```python
from build123d import *

# Parameters (mm, degrees)
CUBE003_W                     = 500
CUBE003_H                     = 500
CUBE003_DEPTH                 = 500
CYLINDER006_R                 = 2.25
CYLINDER006_DEPTH             = 1000
CYLINDER005_R                 = 2.25
CYLINDER005_DEPTH             = 1000
CYLINDER004_R                 = 7.25
CYLINDER004_DEPTH             = 6.5
CYLINDER003_R                 = 7.25
CYLINDER003_DEPTH             = 6.5
GROUP003_PLACEMENT_ANGLE      = 180
CYLINDER002_R                 = 7.25
CYLINDER002_DEPTH             = 6.5
CYLINDER001_R                 = 7.25
CYLINDER001_DEPTH             = 6.5
CYLINDER_R                    = 4
CYLINDER_DEPTH                = 200
CUBE002_W                     = 60
CUBE002_H                     = 21
CUBE002_DEPTH                 = 21
CUBE001_W                     = 30
CUBE001_H                     = 31
CUBE001_DEPTH                 = 26
DIFFERENCE002_PITCH_ANGLE     = 90
DIFFERENCE002_PLACEMENT_ANGLE = 90
REFINELINEAREXTRUDE_R         = 12
REFINELINEAREXTRUDE_R_2       = 1.675
LINEAREXTRUDE_DEPTH           = 20
CUBE_W                        = 42.3
CUBE_H                        = 42.3
CUBE_DEPTH                    = 5
CHAMFER_SIZE                  = 4
CHAMFER001_SIZE               = 1.4
CHAMFER002_SIZE               = 1.4
FILLET_R                      = 5
FILLET001_R                   = 5
FILLET002_R                   = 5
FILLET003_R                   = 5
FILLET004_R                   = 5
FILLET005_R                   = 5


with BuildPart() as cube003:
    # cube003 → cube003 (new body)
    with BuildSketch(Plane(origin=(-250, -510, -250), x_dir=(1, 0, 0), z_dir=(0, 0, 1))):
        with Locations((250, 250)):
            Rectangle(CUBE003_W, CUBE003_H)
    extrude(amount=CUBE003_DEPTH)


with BuildPart() as cylinder006:
    # cylinder006 → cylinder006 (new body)
    with BuildSketch(Plane(origin=(15.5, 500, 0), x_dir=(1, 0, 0), z_dir=(0, -1, 0))):
        Circle(CYLINDER006_R)
    extrude(amount=CYLINDER006_DEPTH)


with BuildPart() as union002:
    # cylinder005 → cylinder005 (new body)
    with BuildSketch(Plane.XZ.offset(-500)):
        Circle(CYLINDER005_R)
    extrude(amount=CYLINDER005_DEPTH)

    # Group005: union cylinder006
    add(cylinder006.part)


with BuildPart() as union002_1:
    # Group005 placement: moved
    add(union002.part.moved(Location((2.25, 0, -15.5))))

    # union002: union cube003
    add(cube003.part)


with BuildPart() as cylinder004:
    # cylinder004 → cylinder004 (new body)
    with BuildSketch(Plane(origin=(15.5, 0, 0), x_dir=(1, 0, 0), z_dir=(0, -1, 0))):
        Circle(CYLINDER004_R)
    extrude(amount=CYLINDER004_DEPTH)


with BuildPart() as group003:
    # cylinder003 → cylinder003 (new body)
    with BuildSketch(Plane.XZ):
        Circle(CYLINDER003_R)
    extrude(amount=CYLINDER003_DEPTH)

    # Group003: union cylinder004
    add(cylinder004.part)


with BuildPart() as group003_1:
    # Group003 placement: moved
    add(group003.part.moved(Location((2.25, 10.5, -15.5))).rotate(Axis((2.25, 10.5, -15.5), (1, 0, 0)), GROUP003_PLACEMENT_ANGLE))


with BuildPart() as cylinder002:
    # cylinder002 → cylinder002 (new body)
    with BuildSketch(Plane(origin=(15.5, 0, 0), x_dir=(1, 0, 0), z_dir=(0, -1, 0))):
        Circle(CYLINDER002_R)
    extrude(amount=CYLINDER002_DEPTH)


with BuildPart() as group004:
    # cylinder001 → cylinder001 (new body)
    with BuildSketch(Plane.XZ):
        Circle(CYLINDER001_R)
    extrude(amount=CYLINDER001_DEPTH)

    # Group002: union cylinder002
    add(cylinder002.part)


with BuildPart() as group004_1:
    # Group002 placement: moved
    add(group004.part.moved(Location((2.25, -10.5, -15.5))))

    # Group004: union Group003
    add(group003_1.part)


with BuildPart() as cylinder:
    # cylinder → cylinder (new body)
    with BuildSketch(Plane(origin=(-100, 15, 13), x_dir=(0, 1, 0), z_dir=(1, 0, 0))):
        Circle(CYLINDER_R)
    extrude(amount=CYLINDER_DEPTH)


with BuildPart() as union:
    # cube002 → cube002 (new body)
    with BuildSketch(Plane(origin=(-30, -10.5, -13), x_dir=(1, 0, 0), z_dir=(0, 0, 1))):
        with Locations((30, 10.5)):
            Rectangle(CUBE002_W, CUBE002_H)
    extrude(amount=CUBE002_DEPTH)

    # union: union cylinder
    add(cylinder.part)


with BuildPart() as difference002:
    # cube001 → cube001 (new body)
    with BuildSketch(Plane(origin=(-15, -15.5, -13), x_dir=(1, 0, 0), z_dir=(0, 0, 1))):
        with Locations((15, 15.5)):
            Rectangle(CUBE001_W, CUBE001_H)
    extrude(amount=CUBE001_DEPTH)

    # difference001: cut union
    add(union.part, mode=Mode.SUBTRACT)


with BuildPart() as difference002_1:
    # difference001 placement: moved
    add(difference002.part.moved(Location((10, 0, -13))))

    # union001: union Group004
    add(group004_1.part)

    # difference002: cut union002
    add(union002_1.part, mode=Mode.SUBTRACT)


with BuildPart() as difference002_2:
    # difference002 pitch: moved
    add(difference002_1.part.rotate(Axis((0, 0, 0), (0, 1, 0)), DIFFERENCE002_PITCH_ANGLE))


with BuildPart() as difference002_3:
    # difference002 placement: moved
    add(difference002_2.part.moved(Location((21.15, 5, 25))).rotate(Axis((21.15, 5, 25), (0, 0, 1)), DIFFERENCE002_PLACEMENT_ANGLE))


with BuildPart() as linearextrude:
    # RefineLinearExtrude → LinearExtrude (new body)
    with BuildSketch(Plane(origin=(0, 0, 0), x_dir=(0, 1, 0), z_dir=(0, 0, 1))):
        Circle(REFINELINEAREXTRUDE_R)
        with Locations((15.5, -15.5)):
            Circle(REFINELINEAREXTRUDE_R_2)
        with Locations((15.5, 15.5)):
            Circle(REFINELINEAREXTRUDE_R_2)
        with Locations((-15.5, 15.5)):
            Circle(REFINELINEAREXTRUDE_R_2)
        with Locations((-15.5, -15.5)):
            Circle(REFINELINEAREXTRUDE_R_2)
    extrude(amount=LINEAREXTRUDE_DEPTH)


with BuildPart() as linearextrude_1:
    # LinearExtrude placement: moved
    add(linearextrude.part.moved(Location((21.15, 21.15, -10))))


with BuildPart() as fillet005:
    # cube → cube (new body)
    with BuildSketch(Plane.XY):
        with Locations((21.15, 21.15)):
            Rectangle(CUBE_W, CUBE_H)
    extrude(amount=CUBE_DEPTH)

    # difference: cut LinearExtrude
    add(linearextrude_1.part, mode=Mode.SUBTRACT)

    # Fusion: union difference002
    add(difference002_3.part)

    # Chamfer
    chamfer_edges = [fillet005.edges().sort_by_distance(p)[0] for p in [
        (20.65, 5, 5),
    ]]
    chamfer(chamfer_edges, length=CHAMFER_SIZE)

    # Chamfer001
    chamfer001_edges = [fillet005.edges().sort_by_distance(p)[0] for p in [
        (4.15, -10.5, 30),
    ]]
    chamfer(chamfer001_edges, length=CHAMFER001_SIZE)

    # Chamfer002
    chamfer002_edges = [fillet005.edges().sort_by_distance(p)[0] for p in [
        (4.15, -10.5, 14.5),
    ]]
    chamfer(chamfer002_edges, length=CHAMFER002_SIZE)

    # Fillet
    fillet_edges = [fillet005.edges().sort_by_distance(p)[0] for p in [
        (8.15, -21, 30),
    ]]
    fillet(fillet_edges, radius=FILLET_R)

    # Fillet001
    fillet001_edges = [fillet005.edges().sort_by_distance(p)[0] for p in [
        (8.15, -21, 0),
    ]]
    fillet(fillet001_edges, radius=FILLET001_R)

    # Fillet002
    fillet002_edges = [fillet005.edges().sort_by_distance(p)[0] for p in [
        (0, 0, 2.5),
    ]]
    fillet(fillet002_edges, radius=FILLET002_R)

    # Fillet003
    fillet003_edges = [fillet005.edges().sort_by_distance(p)[0] for p in [
        (42.3, 0, 2.5),
    ]]
    fillet(fillet003_edges, radius=FILLET003_R)

    # Fillet004
    fillet004_edges = [fillet005.edges().sort_by_distance(p)[0] for p in [
        (42.3, 42.3, 2.5),
    ]]
    fillet(fillet004_edges, radius=FILLET004_R)

    # Fillet005
    fillet005_edges = [fillet005.edges().sort_by_distance(p)[0] for p in [
        (0, 42.3, 2.5),
    ]]
    fillet(fillet005_edges, radius=FILLET005_R)


solid = fillet005.part
```
For this review, take the finished solid that the model builds, in its own axes (mm). A direction names the side the tool comes from. Give positions to 0.01 mm unless a question says otherwise; leave off trailing zeros. Write each loop counter-clockwise with the first axis right and the second up, starting at its lowest first coordinate (ties: lowest second). Pieces come first, ordered by that corner, then holes. Notation, with made-up numbers: M 7,67.5 L 42,67.5 A14 ccw 42,80.5 Z; hole C 15.5,84 d9. An arc over 180 degrees is marked long. Answer as a JSON object with one key per item and string values. Group by question number.
Item 1: For pin 1 Ø2.5 at (x, y) = (5.65, 36.65) entering from +Z; pin 2 Ø13.5 at (x, z) = (19, 20) entering from -Y; pin 3 Ø8 at (x, z) = (33, 16.5) entering from +Y; pin 4 Ø4 at (x, z) = (6.5, 12.5) entering from +Y, all flat-tipped, find the tip position at first contact; note any pin that passes through.
Item 2: For probe 1 along X at (y, z) = (36.65, 3.35) (3 decimals); probe 2 along X at (y, z) = (36, 2); probe 3 along Z at (x, y) = (32, 29), list the stretches that pass through material, from the lowest coordinate up. Write a range as [from, to].
Item 3: Consider section C-C on x = 25. Write out the cut boundary in (y, z).
Item 4: Consider section B-B on y = 21.15. Write out the cut boundary in (x, z).
Item 5: Tool access review of faces 4 (the flat face through (4.15, -10.6, 4.7)), 5 (the flat face through (31.15, 2, 18)), 6 (the flat face through (21, 5, 20)): name each direction out of +Z, -Z, +X, -X, +Y, -Y from which nothing blocks a thin tool from reaching the whole face with its end or side.
Item 6: Consider section D-D on y = 13. Write out the cut boundary in (x, z), plus the area to 3 significant figures.
Item 7: Draft analysis for pull direction Y (two halves, no side actions). For faces 1 (the flat face through (12, 13, 0)), 2 (the flat face through (21, 0, 15)), 3 (the cylindrical face through (13.04, 12.306, 2.465)), state which applies: +Y half, -Y half, draft (parallel to the pull), parting line (faces both ways), or undercut.
Item 8: Consider section A-A on z = 22.75. Write out the cut boundary in (x, y).
Check result:
{
 "1": {"pin 1": "passes through", "pin 2": "stops at y = 0", "pin 3": "stops at y = 5", "pin 4": "stops at y = 1.76"},
 "2": {"probe 1": "x = [0, 3.975], [7.325, 34.975], [38.325, 42.3]", "probe 2": "x = [0, 4.11], [7.19, 35.11], [38.19, 42.3]", "probe 3": "z = [0, 5]"},
 "3": {"outline": "M 0,0 L 9.78,0 L 9.78,5 L 9,5 L 5,9 L 5,30 L 0,30 Z; M 32.52,0 L 42.3,0 L 42.3,5 L 32.52,5 Z"},
 "4": {"outline": "M 0,0 L 9.15,0 L 9.15,5 L 0,5 Z; M 33.15,0 L 42.3,0 L 42.3,5 L 33.15,5 Z"},
 "5": {"face 4": "+Z, -Z, -X, -Y", "face 5": "+Z, +X, +Y, -Y", "face 6": "+Z, +X, -X, +Y"},
 "6": {"outline": "M 0,0 L 12.34,0 L 12.34,5 L 0,5 Z; M 29.96,0 L 42.3,0 L 42.3,5 L 29.96,5 Z", "area": "123 mm^2"},
 "7": {"face 1": "draft", "face 2": "-Y half", "face 3": "undercut"},
 "8": {"outline": "M 4.15,-16.35 L 5.55,-17.75 L 5.65,-17.75 L 5.65,-21 L 10.65,-21 L 10.65,-12.75 L 4.15,-12.75 Z; M 4.15,-8.25 L 10.65,-8.25 L 10.65,0 L 31.15,0 L 31.15,5 L 10.15,5 A4 cw 5.65,1.03 L 5.65,-3.25 L 5.55,-3.25 L 4.15,-4.65 Z"}
}
